Source: three-view drawing plus pictorial views. Frame: mm from the lowest corner of the part. Give positions to 0.01 mm unless a question says otherwise; leave off trailing zeros. Loops run counter-clockwise (first coordinate to the right, second up) from the corner with the lowest first, then second, coordinate; pieces in that order, holes last. Notation, with made-up numbers: (-26.75, 46.25) -> (32.25, 46.25) arc R9 cw to (32.25, 51.25) -> close; hole circle Ø1 at (-22.75, 64.5). An arc over 180 degrees is marked (long way). Put each result on its own line as item: value.
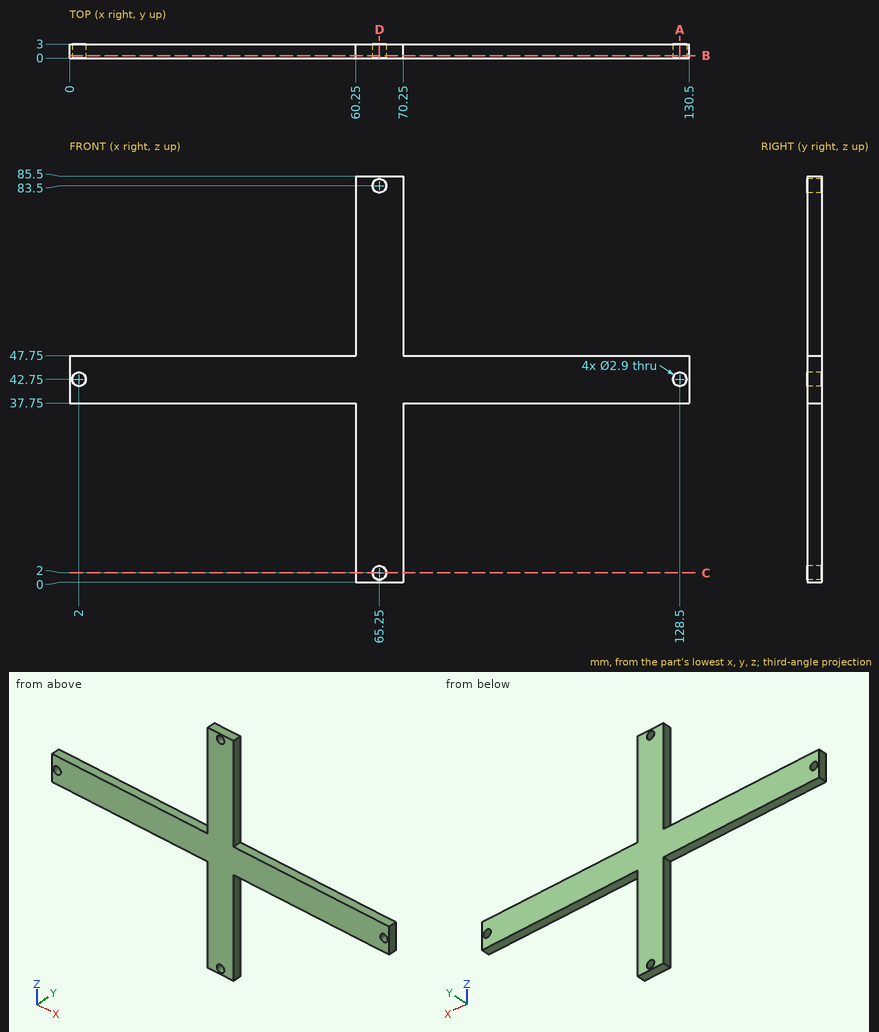
(1) Section C-C on z = 2. Return loops of the section in (x, y), then the cut area to 3 significant figures.
Calculated:
outline: (60.25, 0) -> (63.8, 0) -> (63.8, 3) -> (60.25, 3) -> close; (66.7, 0) -> (70.25, 0) -> (70.25, 3) -> (66.7, 3) -> close
area: 21.3 mm²
(2) First-contact query: P1, Ø1.5, axis at y = 1.5, z = 63, coming from the +X side; P2, Ø0.9, axis at x = 20.5, y = 1.5, coming from the +Z side; P3, Ø1, axis at y = 1.5, z = 63, coming from the -X side; P4, Ø2, axis at x = 66.5, z = 60.5, coming from the -Y side. Flat tips, straight axial feed; report the tip coordinate or a pass-through.
Calculated:
P1: stops at x = 70.25
P2: stops at z = 47.75
P3: stops at x = 60.25
P4: stops at y = 0
(3) Section D-D on x = 65.25. Return loops of the section in (y, z), then the cut area to 3 significant figures.
Calculated:
outline: (0, 0) -> (3, 0) -> (3, 0.55) -> (0, 0.55) -> close; (0, 3.45) -> (3, 3.45) -> (3, 82.05) -> (0, 82.05) -> close; (0, 84.95) -> (3, 84.95) -> (3, 85.5) -> (0, 85.5) -> close
area: 239 mm²
(4) Line query: probe 1 along Z at (x, y) = (65.25, 1.6); probe 2 along X at (y, z) = (1.8, 42.75); probe 3 along Z at (x, y) = (2, 2). Output: solid intervals per line, ascending. Write a range as from..to.
Calculated:
probe 1: z = 0..0.55, 3.45..82.05, 84.95..85.5
probe 2: x = 0..0.55, 3.45..127.05, 129.95..130.5
probe 3: z = 37.75..41.3, 44.2..47.75
(5) Section B-B on y = 0.55. Return loops of the section in (x, z).
Calculated:
outline: (0, 37.75) -> (60.25, 37.75) -> (60.25, 0) -> (70.25, 0) -> (70.25, 37.75) -> (130.5, 37.75) -> (130.5, 47.75) -> (70.25, 47.75) -> (70.25, 85.5) -> (60.25, 85.5) -> (60.25, 47.75) -> (0, 47.75) -> close; hole circle Ø2.9 at (2, 42.75); hole circle Ø2.9 at (65.25, 2); hole circle Ø2.9 at (65.25, 83.5); hole circle Ø2.9 at (128.5, 42.75)
(6) Section A-A on x = 128.5. Return loops of the section in (y, z), then the cut area to 3 significant figures.
Calculated:
outline: (0, 37.75) -> (3, 37.75) -> (3, 41.3) -> (0, 41.3) -> close; (0, 44.2) -> (3, 44.2) -> (3, 47.75) -> (0, 47.75) -> close
area: 21.3 mm²
